```python
from build123d import *

# Parameters (mm, degrees)
SKETCH_1_R      = 5
EXTRUDE_1_DEPTH = 40
EXTRUDE_2_DEPTH = 5
FILLET_1_R      = 1
FILLET_2_R      = 2


with BuildPart() as part:
    # 草图1 → 凸台-拉伸1 (new body)
    with BuildSketch(Plane.XY):
        Circle(SKETCH_1_R)
    extrude(amount=EXTRUDE_1_DEPTH)

    # 草图2 → 凸台-拉伸2 (add)
    with BuildSketch(Plane.XY.offset(40)):
        Polygon((4.330127019, -7.5), (8.660254038, 0), (4.330127019, 7.5), (-4.330127019, 7.5), (-8.660254038, 0), (-4.330127019, -7.5), align=None)
    extrude(amount=EXTRUDE_2_DEPTH)

    # 圆角1
    fillet_1_edges = [part.edges().sort_by_distance(p)[0] for p in [
        (0, -7.5, 45),
        (6.495190528, -3.75, 45),
        (6.495190528, 3.75, 45),
        (0, 7.5, 45),
        (-6.495190528, 3.75, 45),
        (-6.495190528, -3.75, 45),
    ]]
    fillet(fillet_1_edges, radius=FILLET_1_R)

    # 圆角2
    fillet_2_edges = [part.edges().sort_by_distance(p)[0] for p in [
        (-5, 0, 0),
    ]]
    fillet(fillet_2_edges, radius=FILLET_2_R)


solid = part.part
```
Model file for the job. Use its own axes, mm. A direction names the side the tool comes from. Round coordinates to 2 decimals unless told otherwise and drop trailing zeros. Order: outer loops, then holes, each group sorted by start corner. A loop starts at its lowest first (then second) coordinate and runs counter-clockwise, first axis right, second up. Notation, with made-up numbers: (28.25, -35.75) -> (45.25, -35.75) arc R29 ccw to (45.25, -6.75) -> close; hole circle Ø3 at (2.5, 53). An arc over 180 degrees is marked (long way). Use one line per item in the form item = value.
Item 1: Cut at A-A, the plane z = 42. Write the cut outline in (x, y).
Returned:
outline = (-8.66, 0) -> (-4.33, -7.5) -> (4.33, -7.5) -> (8.66, 0) -> (4.33, 7.5) -> (-4.33, 7.5) -> close
Item 2: Drill centre lines: line 1 (Z direction, x = 4.5, y = 3); line 2 (Y direction, x = 0.25, z = 35.5); line 3 (X direction, y = -3, z = 32.5). Where is each one in solid material? Low to high.
Returned:
line_1 = 40 to 45
line_2 = -4.99 to 4.99
line_3 = -4 to 4
Item 3: Cut at B-B, the plane x = 0. Write the cut outline in (y, z).
Returned:
outline = (-7.5, 40) -> (-5, 40) -> (-5, 2) arc R2 ccw to (-3, 0) -> (3, 0) arc R2 ccw to (5, 2) -> (5, 40) -> (7.5, 40) -> (7.5, 44) arc R1 ccw to (6.5, 45) -> (-6.5, 45) arc R1 ccw to (-7.5, 44) -> close
Item 4: Tool access for faces 1 (the face through (6.22, 3.66, 44.7)), 2 (the face through (2, 5, 40)): list every direction of +Z, -Z, +X, -X, +Y, -Y with a clear straight run to the whole face (end or side of a thin tool).
Returned:
face_1 = +Z, +X, +Y
face_2 = -Z
Item 5: Flat gauge pins, fed straight in: pin 1 Ø3 at (x, y) = (-5.5, 4) entering from +Z; pin 2 Ø4 at (x, z) = (0.5, 29.5) entering from -Y; pin 3 Ø2 at (y, z) = (-5, 26) entering from +X. Where does each tip first touch, or does it go through?
Returned:
pin_1 = 45
pin_2 = -5
pin_3 = 3
